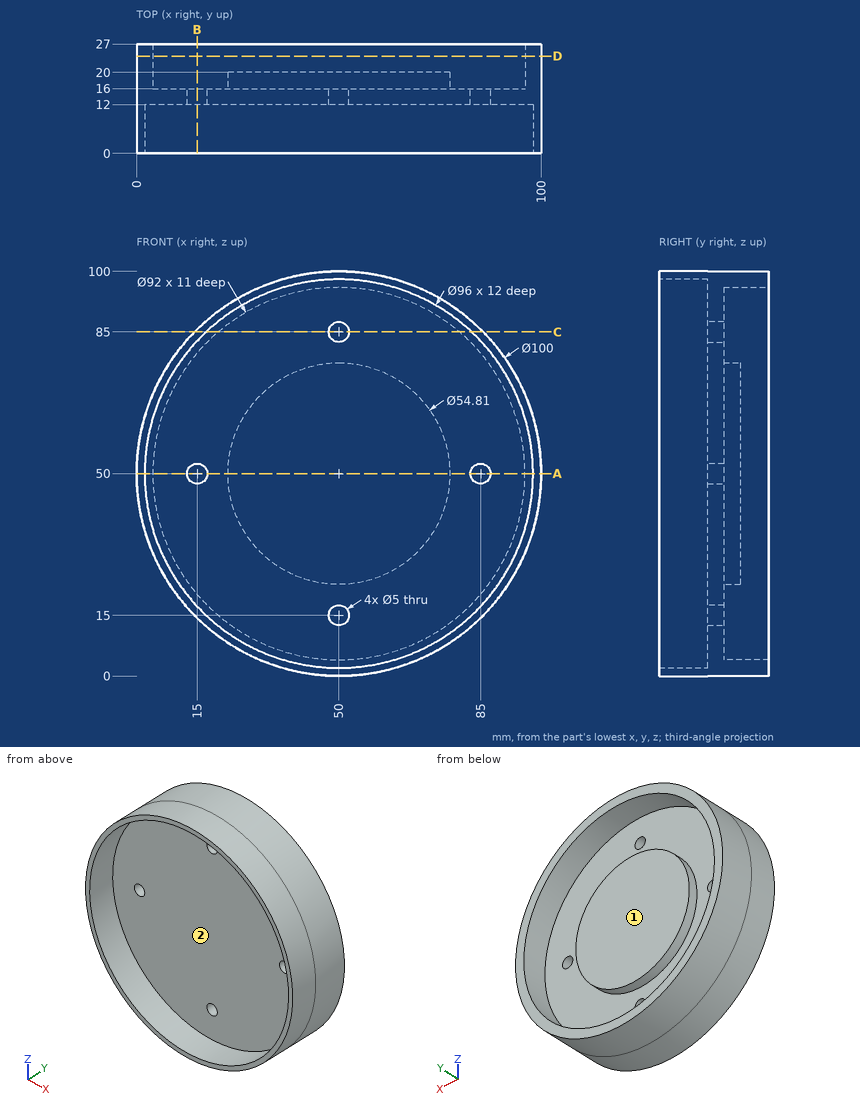
Drawing for the job (mm, zero at the part's lowest x, y, z). A direction names the side the tool comes from. Give positions to 0.01 mm unless a question says otherwise; leave off trailing zeros. Loops run counter-clockwise (first coordinate to the right, second up) from the corner with the lowest first, then second, coordinate; pieces in that order, holes last.
1) Band-saw the part on A-A on z = 50. List the corners of the cut face in (x, y) (3 decimals), then the cut area to 3 significant figures.
Values follow:
outline: (0, 0) - (2, 0) - (2, 12) - (12.5, 12) - (12.5, 16) - (4, 16) - (4, 27) - (0, 27) - close; (17.5, 12) - (82.5, 12) - (82.5, 16) - (77.405, 16) - (77.405, 20) - (22.595, 20) - (22.595, 16) - (17.5, 16) - close; (87.5, 12) - (98, 12) - (98, 0) - (100, 0) - (100, 27) - (96, 27) - (96, 16) - (87.5, 16) - close
area: 715 mm2
2) Band-saw the part on C-C on z = 85. List the corners of the cut face in (x, y), then the cut area to 3 significant figures.
Values follow:
outline: (14.29, 0) - (17.15, 0) - (17.15, 12) - (47.5, 12) - (47.5, 16) - (20.15, 16) - (20.15, 27) - (14.29, 27) - close; (52.5, 12) - (82.85, 12) - (82.85, 0) - (85.71, 0) - (85.71, 27) - (79.85, 27) - (79.85, 16) - (52.5, 16) - close
area: 463 mm2
3) Band-saw the part on B-B on x = 15. List the corners of the cut face in (y, z), then the cut area to 3 significant figures.
Values follow:
outline: (0, 14.29) - (27, 14.29) - (27, 20.15) - (16, 20.15) - (16, 47.5) - (12, 47.5) - (12, 17.15) - (0, 17.15) - close; (0, 82.85) - (12, 82.85) - (12, 52.5) - (16, 52.5) - (16, 79.85) - (27, 79.85) - (27, 85.71) - (0, 85.71) - close
area: 463 mm2
4) 3-axis set-ups, long thin cutter, end or side, ignore diameter. For the marked faces 1 and 2: which of +Z, -Z, +X, -X, +Y, -Y reach the whole face in a straight line?
Values follow:
face 1: +Y
face 2: -Y
5) Drop flat-ended pins along their axis: P1, Ø10, axis at y = 16, z = 10.5, coming from the -X side; P2, Ø6, axis at x = 66.5, z = 16.5, coming from the -Y side; P3, Ø1.5, axis at x = 45, z = 39, coming from the +Y side. Give the stop position or say it passes through.
Values follow:
P1: stops at x = 13.81
P2: stops at y = 12
P3: stops at y = 20
6) Probe line 1 along X through (y, z) = (18.5, 50) (3 decimals); line 2 along X through (y, z) = (13.3, 50); line 3 along Z through (x, y) = (63.5, 17.25). List the from-to ranges inside material, lowest first.
Values follow:
line 1: x = 0 to 4, 22.595 to 77.405, 96 to 100
line 2: x = 0 to 12.5, 17.5 to 82.5, 87.5 to 100
line 3: z = 1.86 to 6.03, 26.15 to 73.85, 93.97 to 98.14
7) Band-saw the part on D-D on y = 24. List the corners of the cut face in (x, z), then the cut area to 3 significant figures.
Values follow:
outline: circle Ø100 at (50, 50); hole circle Ø92 at (50, 50)
area: 1,210 mm2
